Model file for the job. Use its own axes, mm. A direction names the side the tool comes from. Give positions to 0.01 mm unless a question says otherwise; leave off trailing zeros. Order: outer loops, then holes, each group sorted by start corner. A loop starts at its lowest first (then second) coordinate and runs counter-clockwise, first axis right, second up. Notation, with made-up numbers: M 77.25,36 L 117.25,36 A13 ccw 117.25,58 Z; hole C 48.25,73 d6. An arc over 180 degrees is marked long. Return JSON: item names as keys, results as strings. Group by question number.
1. Slice it at D-D on z = 78.5. List the corners of the cut face in (x, y).
2. Pin check, flat tips, straight feed: pin 1 (6 mm diameter, centred on x = -7, z = -38.5, fed in from +Y); pin 2 (4 mm diameter, centred on x = -3, y = 6, fed in from -Z); pin 3 (5 mm diameter, centred on x = 11, y = 3.5, fed in from +Z). Stop position of each tip, or through.
3. Two-plate mould, pull along X, no slides. Class faces 1 (the face through (0, 1.6, -1)), 2 (the face through (11.79, 0.81, 89.71)), 3 (the face through (-2.346, 8.995, -58.247)): released by +X, released by -X, zero draft, split by the parting line, or undercut.
4. 3-axis set-ups, long thin cutter, end or side, ignore diameter. For faces 4 (the face through (11.79, 0.81, -86.29)), 5 (the face through (-3.841, 8.995, 81.733)): which of +Z, -Z, +X, -X, +Y, -Y reach the whole face in a straight line?
5. Wall check: probe 1 along Z at (x, y) = (-4, 13.5); probe 2 along X at (y, z) = (0.6, 88); probe 3 along X at (y, z) = (0.8, -73). Give the ranges that are in metal, low to high. Write a range as [from, to].
6. Slice it at C-C on y = 10.25. List the corners of the cut face in (x, z).
7. Slice it at B-B on x = 12.5. List the corners of the cut face in (y, z), then the cut area to 3 significant figures.
8. Slice it at A-A on z = -38.5. List the corners of the cut face in (x, y).
from build123d import *

# Parameters (mm, degrees)
SKETCH1_W           = 33
SKETCH1_H           = 184
BOSS_EXTRUDE1_DEPTH = 1.6
SKETCH2_R           = 1.85
CUT_EXTRUDE1_DEPTH  = 94.481602468
SKETCH3_R           = 3.5
BOSS_EXTRUDE2_DEPTH = 15
SKETCH4_W           = 17
SKETCH4_H           = 12
CUT_EXTRUDE2_DEPTH  = 95.663879067


with BuildPart() as part:
    # Sketch1 → Boss-Extrude1 (new body)
    with BuildSketch(Plane(origin=(0, 0, 0), x_dir=(1, 0, 0), z_dir=(0, 1, 0))):
        Rectangle(SKETCH1_W, SKETCH1_H)
    extrude(amount=BOSS_EXTRUDE1_DEPTH)

    # Sketch2 → Cut-Extrude1 (cut, through all)
    with BuildSketch(Plane(origin=(0, 1.6, 0), x_dir=(1, 0, 0), z_dir=(0, 1, 0))):
        with Locations(Location((-12.5, 73, 0), (0, 0, 270))):
            Circle(SKETCH2_R)
        with Locations(Location((12.5, 88, 0), (0, 0, 270))):
            Circle(SKETCH2_R)
        with Locations(Location((12.5, -88, 0), (0, 0, 270))):
            Circle(SKETCH2_R)
    extrude(amount=-CUT_EXTRUDE1_DEPTH, mode=Mode.SUBTRACT)

    # Sketch3 → Boss-Extrude2 (add)
    with BuildSketch(Plane(origin=(0, 1.6, 0), x_dir=(1, 0, 0), z_dir=(0, 1, 0))):
        with Locations(Location((-2.5, 84, 0), (0, 0, 270))):
            Circle(SKETCH3_R)
        with Locations(Location((-2.5, 54.75, 0), (0, 0, 270))):
            Circle(SKETCH3_R)
        with Locations(Location((-2.5, 20.75, 0), (0, 0, 270))):
            Circle(SKETCH3_R)
        with Locations(Location((-2.5, -78.5, 0), (0, 0, 270))):
            Circle(SKETCH3_R)
    extrude(amount=BOSS_EXTRUDE2_DEPTH)

    # Sketch4 → Cut-Extrude2 (cut, through all)
    with BuildSketch(Plane(origin=(0, 1.6, 0), x_dir=(1, 0, 0), z_dir=(0, 1, 0))):
        with Locations((-1.5, 35)):
            Rectangle(SKETCH4_W, SKETCH4_H)
    extrude(amount=-CUT_EXTRUDE2_DEPTH, mode=Mode.SUBTRACT)


solid = part.part
Result:
{
 "1": {"outline": "M -16.5,0 L 16.5,0 L 16.5,1.6 L 1,1.6 L 1,16.6 L -6,16.6 L -6,1.6 L -16.5,1.6 Z"},
 "2": {"pin 1": "stops at y = 1.6", "pin 2": "stops at z = -87.5", "pin 3": "stops at z = 92"},
 "3": {"face 1": "zero draft", "face 2": "undercut", "face 3": "split by the parting line"},
 "4": {"face 4": "+Y, -Y", "face 5": "+Y"},
 "5": {"probe 1": "z = [-87.16, -80.84], [-57.91, -51.59], [-23.91, -17.59], [75.34, 81.66]", "probe 2": "x = [-16.5, 10.65], [14.35, 16.5]", "probe 3": "x = [-16.5, -14.35], [-10.65, 16.5]"},
 "6": {"outline": "C -2.5,-84 d7; C -2.5,-54.75 d7; C -2.5,-20.75 d7; C -2.5,78.5 d7"},
 "7": {"outline": "M 0,-92 L 1.6,-92 L 1.6,-89.85 L 0,-89.85 Z; M 0,-86.15 L 1.6,-86.15 L 1.6,86.15 L 0,86.15 Z; M 0,89.85 L 1.6,89.85 L 1.6,92 L 0,92 Z", "area": "283 mm2"},
 "8": {"outline": "M -16.5,0 L -10,0 L -10,1.6 L -16.5,1.6 Z; M 7,0 L 16.5,0 L 16.5,1.6 L 7,1.6 Z"}
}
